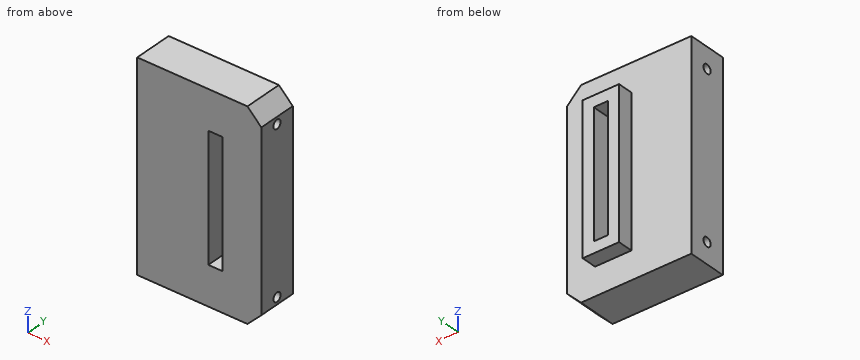
from build123d import *

# Parameters (mm, degrees)
SKETCH1_W           = 44.7
SKETCH1_H           = 73
SKETCH1_W_2         = 5.1
SKETCH1_H_2         = 45
BOSS_EXTRUDE1_DEPTH = 14
CUT_EXTRUDE1_REACH  = 46.7
SKETCH2_R           = 1.6
SKETCH3_W           = 13.1
SKETCH3_H           = 53
SKETCH3_W_2         = 5.1
SKETCH3_H_2         = 45
BOSS_EXTRUDE2_DEPTH = 5.5
CUT_EXTRUDE2_REACH  = 16


with BuildPart() as part:
    # Sketch1 → Boss-Extrude1 (new body)
    with BuildSketch(Plane(origin=(0, 0, 0), x_dir=(1, 0, 0), z_dir=(0, 1, 0))):
        with Locations((0.284066801, -8.539694425)):
            Rectangle(SKETCH1_W, SKETCH1_H)
        with Locations((6.084066801, -8.539694425)):
            Rectangle(SKETCH1_W_2, SKETCH1_H_2, mode=Mode.SUBTRACT)
    extrude(amount=BOSS_EXTRUDE1_DEPTH)

    # Sketch2 → Cut-Extrude1 (cut, up to next)
    with BuildSketch(Plane(origin=(22.634066801, 0, 0), x_dir=(0, 0, -1), z_dir=(1, 0, 0)), mode=Mode.PRIVATE) as cut_extrude1_sk1:
        with Locations((-37.539694425, 7)):
            Circle(SKETCH2_R)
    cut_extrude1_tool1 = extrude(cut_extrude1_sk1.sketch, amount=-CUT_EXTRUDE1_REACH, mode=Mode.PRIVATE) & part.part
    add(cut_extrude1_tool1.solids().sort_by_distance((22.634067, 7, 37.539694))[0], mode=Mode.SUBTRACT)
    # Sketch2 → Cut-Extrude1 (cut, up to next)
    with BuildSketch(Plane(origin=(22.634066801, 0, 0), x_dir=(0, 0, -1), z_dir=(1, 0, 0)), mode=Mode.PRIVATE) as cut_extrude1_sk2:
        with Locations((20.460305575, 7)):
            Circle(SKETCH2_R)
    cut_extrude1_tool2 = extrude(cut_extrude1_sk2.sketch, amount=-CUT_EXTRUDE1_REACH, mode=Mode.PRIVATE) & part.part
    add(cut_extrude1_tool2.solids().sort_by_distance((22.634067, 7, -20.460306))[0], mode=Mode.SUBTRACT)

    # Sketch3 → Boss-Extrude2 (add)
    with BuildSketch(Plane(origin=(0, 14, 0), x_dir=(1, 0, 0), z_dir=(0, 1, 0))):
        with Locations((6.084066801, -8.539694425)):
            Rectangle(SKETCH3_W, SKETCH3_H)
        with Locations((6.084066801, -8.539694425)):
            Rectangle(SKETCH3_W_2, SKETCH3_H_2, mode=Mode.SUBTRACT)
    extrude(amount=BOSS_EXTRUDE2_DEPTH)

    # Sketch4 → Cut-Extrude2 (cut, up to next)
    with BuildSketch(Plane(origin=(0, 14, 0), x_dir=(1, 0, 0), z_dir=(0, 1, 0)), mode=Mode.PRIVATE) as cut_extrude2_sk1:
        Polygon((17.634066801, 27.960305575), (22.634066801, 22.960305575), (22.634066801, 27.960305575), align=None)
    cut_extrude2_tool1 = extrude(cut_extrude2_sk1.sketch, amount=-CUT_EXTRUDE2_REACH, mode=Mode.PRIVATE) & part.part
    add(cut_extrude2_tool1.solids().sort_by_distance((20.9674, 14, -26.293639))[0], mode=Mode.SUBTRACT)
    # Sketch4 → Cut-Extrude2 (cut, up to next)
    with BuildSketch(Plane(origin=(0, 14, 0), x_dir=(1, 0, 0), z_dir=(0, 1, 0)), mode=Mode.PRIVATE) as cut_extrude2_sk2:
        Polygon((17.634066801, -45.039694425), (22.634066801, -40.039694425), (22.634066801, -45.039694425), align=None)
    cut_extrude2_tool2 = extrude(cut_extrude2_sk2.sketch, amount=-CUT_EXTRUDE2_REACH, mode=Mode.PRIVATE) & part.part
    add(cut_extrude2_tool2.solids().sort_by_distance((20.9674, 14, 43.373028))[0], mode=Mode.SUBTRACT)


solid = part.part
Work out the finished part from the listing and answer in its coordinate system (mm). Round coordinates to 2 decimals unless told otherwise and drop trailing zeros. Order: outer loops, then holes, each group sorted by start corner. A loop starts at its lowest first (then second) coordinate and runs counter-clockwise, first axis right, second up. Notation, with made-up numbers: M 86,73 L 116,73 A13 ccw 116,78 Z; hole C 88.5,-11 d8. An arc over 180 degrees is marked long. Put each result on its own line as item: value. Start each with the question number.
Q1. Straight lines are drawn through the part: L1, parallel to Z at x = 8.5, y = 10.25; L2, parallel to Z at x = -18.5, y = 8; L3, parallel to X at y = 9.75, z = -12. For each, find the intervals that lie inside material, in ascending order. Write a range as [from, to].
Q2. Section A-A, the plane y = 7 is taken. Write down the section's boundary in (x, z).
Q3. Section B-B, the plane z = -20.5 is taken. Write down the section's boundary in (x, y).
Q4. Section D-D, the plane x = 15.5 is taken. Write down the section's boundary in (y, z).
Q5. Flat-ended cylindrical pins translate along their axes: pin 1 (1.6 mm diameter, centred on y = 15.5, z = 6.5, fed in from -X); pin 2 (1.5 mm diameter, centred on x = -7.5, z = 19, fed in from +Y); pin 3 (3 mm diameter, centred on y = 16, z = 13, fed in from +X). Find the tip coordinate at first contact, or state that the pin passes through.
Q6. Section C-C, the plane z = 33 is taken. Write down the section's boundary in (x, y).
Findings below:
1. L1: z = [-27.96, -13.96], [31.04, 45.04]
1. L2: z = [-27.96, -21.71], [-19.21, 36.29], [38.79, 45.04]
1. L3: x = [-22.07, 3.53], [8.63, 22.63]
2. outline: M -22.07,-27.96 L 17.63,-27.96 L 22.63,-22.96 L 22.63,-22.06 L -22.07,-22.06 Z; M -22.07,-18.86 L 22.63,-18.86 L 22.63,35.94 L -22.07,35.94 Z; M -22.07,39.14 L 22.63,39.14 L 22.63,40.04 L 17.63,45.04 L -22.07,45.04 Z; hole M 3.53,-13.96 L 8.63,-13.96 L 8.63,31.04 L 3.53,31.04 Z
3. outline: M -22.07,0 L 22.63,0 L 22.63,5.4 L -22.07,5.4 Z; M -22.07,8.6 L 22.63,8.6 L 22.63,14 L -22.07,14 Z
4. outline: M 0,-27.96 L 14,-27.96 L 14,45.04 L 0,45.04 Z; hole C 7,-20.46 d3.2; hole C 7,37.54 d3.2
5. pin 1: stops at x = -0.47
5. pin 2: stops at y = 14
5. pin 3: stops at x = 12.63
6. outline: M -22.07,0 L 22.63,0 L 22.63,14 L 12.63,14 L 12.63,19.5 L -0.47,19.5 L -0.47,14 L -22.07,14 Z
